```python
from build123d import *

# Parameters (mm, degrees)
BOSS_EXTRUDE1_DEPTH = 12
SKETCH3_W           = 25
SKETCH3_H           = 25
CUT_EXTRUDE1_DEPTH  = 7
SKETCH4_W           = 18
SKETCH4_H           = 25
SKETCH4_R           = 2.6
BOSS_EXTRUDE2_DEPTH = 5
CHAMFER1_SIZE       = 2
CUT_EXTRUDE2_DEPTH  = 5
FILLET1_R           = 5
FILLET2_R           = 0.5


with BuildPart() as part:
    # Sketch1 → Boss-Extrude1 (new body)
    with BuildSketch(Plane.XY):
        with BuildLine():
            Line((-22.5, 12.5), (-28.5, 6.5))
            Line((-28.5, 6.5), (-28.5, -1.5))
            Line((-28.5, -1.5), (-17.5, -12.5))
            Line((-17.5, -12.5), (28.5, -12.5))
            Line((28.5, -12.5), (28.5, 12.5))
            Line((28.5, 12.5), (-3.5, 12.5))
            Line((-3.5, 12.5), (-3.5, 6))
            Line((-3.5, 6), (-13.382383367, 6))
            ThreePointArc((-13.382383367, 6), (-23.330458604, -1.386729946), (-13.985855563, 6.75))
            Line((-13.985855563, 6.75), (-4.25, 6.75))
            Line((-4.25, 6.75), (-4.25, 12.5))
            Line((-4.25, 12.5), (-5.7, 12.5))
            Line((-5.7, 12.5), (-22.5, 12.5))
        make_face()
    extrude(amount=BOSS_EXTRUDE1_DEPTH)

    # Sketch3 → Cut-Extrude1 (cut)
    with BuildSketch(Plane.XY.offset(12)):
        with Locations((16, 0)):
            Rectangle(SKETCH3_W, SKETCH3_H)
    extrude(amount=-CUT_EXTRUDE1_DEPTH, mode=Mode.SUBTRACT)

    # Sketch4 → Boss-Extrude2 (add)
    with BuildSketch(Plane(origin=(3.5, 0, 0), x_dir=(0, 0, -1), z_dir=(1, 0, 0))):
        with Locations((-21, 0)):
            Rectangle(SKETCH4_W, SKETCH4_H)
        with Locations(Location((-20, -5, 0), (0, 0, 90))):
            Circle(SKETCH4_R, mode=Mode.SUBTRACT)
    extrude(amount=-BOSS_EXTRUDE2_DEPTH)

    # Chamfer1
    chamfer1_edges = [part.edges().sort_by_distance(p)[0] for p in [
        (-1.5, 0, 12),
    ]]
    chamfer(chamfer1_edges, length=CHAMFER1_SIZE)

    # Sketch5 → Cut-Extrude2 (cut)
    with BuildSketch(Plane.XY.offset(5)):
        with BuildLine():
            Line((15.9, 2.5), (15.9, 12.5))
            Line((15.9, 12.5), (21.1, 12.5))
            Line((21.1, 12.5), (21.1, 2.5))
            ThreePointArc((21.1, 2.5), (18.5, -0.1), (15.9, 2.5))
        make_face()
    extrude(amount=-CUT_EXTRUDE2_DEPTH, mode=Mode.SUBTRACT)

    # Fillet1
    fillet1_edges = [part.edges().sort_by_distance(p)[0] for p in [
        (-17.5, -12.5, 6),
        (-28.5, -1.5, 6),
        (-28.5, 6.5, 6),
        (-22.5, 12.5, 6),
    ]]
    fillet(fillet1_edges, radius=FILLET1_R)

    # Fillet2
    fillet2_edges = [part.edges().sort_by_distance(p)[0] for p in [
        (-13.985855563, 6.75, 6),
        (-13.382383367, 6, 6),
        (28.5, 12.5, 2.5),
        (28.5, -12.5, 2.5),
        (3.5, -12.5, 17.5),
        (3.5, 12.5, 17.5),
        (-1.5, -12.5, 22),
        (-1.5, 12.5, 22),
        (15.9, 12.5, 2.5),
        (21.1, 12.5, 2.5),
    ]]
    fillet(fillet2_edges, radius=FILLET2_R)

    # Sketch6 → Cut-Revolve1 (revolve, cut)
    with BuildSketch(Plane(origin=(0, 0, 6), x_dir=(-1, 0, 0), z_dir=(0, 0, -1)), mode=Mode.PRIVATE) as cut_revolve1_sk:
        Polygon((8.5, 12.5), (10.25, 12.5), (10.25, -7.5), (10.85, -7.5), (10.85, -12), (11, -12), (11, -12.5), (8.5, -12.5), align=None)
    revolve(cut_revolve1_sk.sketch.rotate(Axis((-8.5, 12.5, 6), (0, -1, 0)), 270), axis=Axis((-8.5, 12.5, 6), (0, -1, 0)), mode=Mode.SUBTRACT)


solid = part.part
```
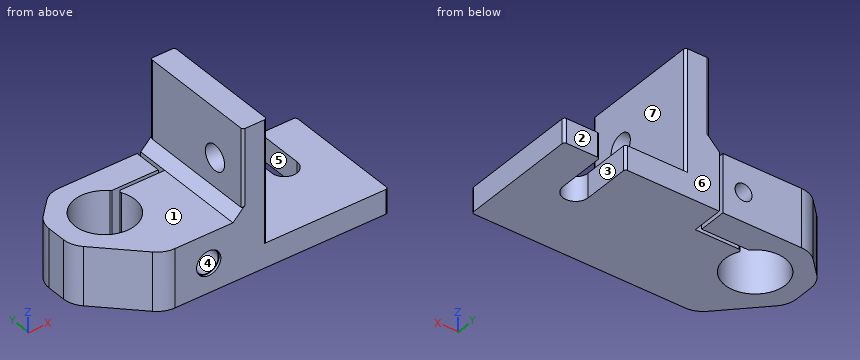
Verification items for the finished model (mm, model axes). Face numbers are marked on the shaded views. A direction names the side the tool comes from. Coordinates: 2 decimals unless noted, no trailing zeros. Write each loop counter-clockwise with the first axis right and the second up, starting at its lowest first coordinate (ties: lowest second). Pieces come first, ordered by that corner, then holes. Notation, with made-up numbers: (-2, 58.25) - (36, 58.25) arc R25 ccw to (36, 89.25) - close; hole circle Ø3 at (86.25, 50). An arc over 180 degrees is marked (long way). One line per question, with ' | ' between items. Start each with the question number.
1. Section check D-D (z = 28). Enter the section's corners in (x, y).
2. Gauge pin test, flat ends, axial feed: P1, Ø1, axis at y = 6, z = 9.5, coming from the +X side; P2, Ø4, axis at x = 14.5, y = 3.5, coming from the +Z side; P3, Ø4, axis at x = -8.5, z = 6, coming from the -Y side. Record the tip position at first contact, or that the pin passes through.
3. Material ranges on line 1 along Z through (x, y) = (-8.5, 9.8); line 2 along X through (y, z) = (2.5, 4.75); line 3 along X through (y, z) = (10, 2.25), recorded low to high.
4. Draft check along X on the marked faces 5, 6 and 7. Enter one of: released by +X, released by -X, zero draft, split by the parting line, or undercut.
5. Access from +Z, -Z, +X, -X, +Y, -Y to the whole of each face (thin tool, end or side, straight path). Record for the marked faces 1, 2, 3 and 4.
6. Section check A-A (y = -5). Enter the section's corners in (x, z).
7. Section check B-B (z = 21). Enter the section's corners in (x, y).
8. Section check C-C (x = -8.5). Enter the section's corners in (y, z), plus the area to 3 significant figures.
Computed values:
1) outline: (-1.5, -12) arc R0.5 ccw to (-1, -12.5) - (3, -12.5) arc R0.5 ccw to (3.5, -12) - (3.5, 12) arc R0.5 ccw to (3, 12.5) - (-1, 12.5) arc R0.5 ccw to (-1.5, 12) - close
2) P1: x = 3.5 | P2: z = 5 | P3: y = -7.5
3) line 1: 0 to 4.25, 7.75 to 12 | line 2: -28.5 to -24.7, -12.3 to -9.72, -7.28 to 15.9, 21.1 to 28.5 | line 3: -25 to -4.25, -3.5 to 15.9, 21.1 to 28.5
4) face 5: undercut | face 6: zero draft | face 7: released by +X
5) face 1: +Z, -X, +Y, -Y | face 2: +Z, -Z, +X, -X, +Y | face 3: +Z, -Z, +Y | face 4: -Y
6) outline: (-25, 0) - (28.5, 0) - (28.5, 5) - (3.5, 5) - (3.5, 17.4) - (-1.5, 17.4) - (-1.5, 14) - (-3.5, 12) - (-25, 12) - close; (-1.5, 22.6) - (3.5, 22.6) - (3.5, 30) - (-1.5, 30) - close; hole circle Ø3.5 at (-8.5, 6)
7) outline: (-1.5, -12) arc R0.5 ccw to (-1, -12.5) - (3, -12.5) arc R0.5 ccw to (3.5, -12) - (3.5, -7.4) - (-1.5, -7.4) - close; (-1.5, -2.6) - (3.5, -2.6) - (3.5, 12) arc R0.5 ccw to (3, 12.5) - (-1, 12.5) arc R0.5 ccw to (-1.5, 12) - close
8) outline: (-12.5, 0) - (6, 0) - (6, 4.25) - (-7.5, 4.25) - (-7.5, 3.65) - (-12, 3.65) - (-12, 3.5) - (-12.5, 3.5) - close; (-12.5, 8.5) - (-12, 8.5) - (-12, 8.35) - (-7.5, 8.35) - (-7.5, 7.75) - (6, 7.75) - (6, 12) - (-12.5, 12) - close; (6.75, 0) - (12.5, 0) - (12.5, 4.25) - (6.75, 4.25) - close; (6.75, 7.75) - (12.5, 7.75) - (12.5, 12) - (6.75, 12) - close | area: 200 mm²
